from build123d import *

# Parameters (mm, degrees)
SALIENTE_EXTRUIR1_DEPTH = 8
CROQUIS2_R              = 10
CORTAR_EXTRUIR1_DEPTH   = 29.91366459
REDONDEO1_R             = 2
CROQUIS3_R              = 1.5
CORTAR_EXTRUIR2_DEPTH   = 30.159046624


with BuildPart() as part:
    # Croquis1 → Saliente-Extruir1 (new body)
    with BuildSketch(Plane.XY):
        with BuildLine():
            Line((-24, -0.5), (-13.99106858, -0.5))
            ThreePointArc((-13.99106858, -0.5), (0, 14), (13.99106858, -0.5))
            Line((13.99106858, -0.5), (24, -0.5))
            Line((24, -0.5), (24, -4.5))
            Line((24, -4.5), (13.257073584, -4.5))
            ThreePointArc((13.257073584, -4.5), (0, -14), (-13.257073584, -4.5))
            Line((-13.257073584, -4.5), (-24, -4.5))
            Line((-24, -4.5), (-24, -0.5))
        make_face()
    extrude(amount=SALIENTE_EXTRUIR1_DEPTH)

    # Croquis2 → Cortar-Extruir1 (cut, through all)
    with BuildSketch(Plane.XY.offset(8)):
        Circle(CROQUIS2_R)
    extrude(amount=-CORTAR_EXTRUIR1_DEPTH, mode=Mode.SUBTRACT)

    # Redondeo1
    redondeo1_edges = [part.edges().sort_by_distance(p)[0] for p in [
        (24, -2.5, 8),
        (-24, -2.5, 8),
        (-24, -2.5, 0),
        (24, -2.5, 0),
    ]]
    fillet(redondeo1_edges, radius=REDONDEO1_R)

    # Croquis3 → Cortar-Extruir2 (cut, through all)
    with BuildSketch(Plane(origin=(0, -0.5, 0), x_dir=(1, 0, 0), z_dir=(0, 1, 0))):
        with Locations(Location((-17.99553429, -4, 0), (0, 0, 270))):
            Circle(CROQUIS3_R)
        with Locations(Location((17.99553429, -4, 0), (0, 0, 270))):
            Circle(CROQUIS3_R)
    extrude(amount=-CORTAR_EXTRUIR2_DEPTH, mode=Mode.SUBTRACT)


solid = part.part
CAD build for the part. Positions are in the model's coordinates, mm. A direction names the side the tool comes from. Round coordinates to 2 decimals unless told otherwise and drop trailing zeros. Loops run counter-clockwise (first coordinate to the right, second up) from the corner with the lowest first, then second, coordinate; pieces in that order, holes last.
(1) Cut at B-B (x = 0). Give the cut face in (y, z), plus the area to 3 significant figures.
(2) Two-plate mould, pull along Z, no slides. Class faces 1 (the cylindrical face through (-19.326, -2.472, 4.692)), 2 (the cylindrical face through (23.4, -2.53, 0.57)), 3 (the flat face through (0.1, -10.3, 8)): +Z half, -Z half, draft (parallel to the pull), parting line (faces both ways), or undercut.
(3) Which spindle directions (+Z, -Z, +X, -X, +Y, -Y) get a long thin tool onto all of the face, cutting with end or side? Do faces 4 (the flat face through (-20, -4.5, 4)), 5 (the flat face through (20, -0.5, 4)), 6 (the flat face through (20, -4.5, 4)). Say none if no direction does.
(4) Cut at A-A (z = 4). Give the cut face in (x, y), plus the area to 3 significant figures.
(5) Drop flat-ended pins along their axis: pin 1 (3 mm diameter, centred on x = -1.5, z = 2.5, fed in from -Y); pin 2 (2 mm diameter, centred on x = 8.5, z = 1, fed in from +Y); pin 3 (2.5 mm diameter, centred on x = -17, z = 4, fed in from +Y); pin 4 (2 mm diameter, centred on y = -11, z = 6, fed in from -X). Give the stop position or say it passes through.
(6) Cut at D-D (x = 15.5). Give the cut face in (y, z), plus the area to 3 significant figures.
(7) Wall check: line 1 along X through (y, z) = (-2.45, 4); line 2 along X through (y, z) = (-3.25, 4); line 3 along Y through (x, z) = (20, 5). Give the ranges that are in metal, low to high.
Findings below:
1. outline: (-14, 0) - (-10, 0) - (-10, 8) - (-14, 8) - close; (10, 0) - (14, 0) - (14, 8) - (10, 8) - close
1. area: 64.0 mm2
2. face 1: undercut
2. face 2: -Z half
2. face 3: +Z half
3. face 4: +Z, -Z, -X, -Y
3. face 5: +Z, -Z, +X, +Y
3. face 6: +Z, -Z, +X, -Y
4. outline: (-24, -4.5) - (-19.5, -4.5) - (-19.5, -0.5) - (-24, -0.5) - close; (-16.5, -4.5) - (-13.26, -4.5) arc R14 ccw to (13.26, -4.5) - (16.5, -4.5) - (16.5, -0.5) - (13.99, -0.5) arc R14 ccw (long way) to (-13.99, -0.5) - (-16.5, -0.5) - close; (19.5, -4.5) - (24, -4.5) - (24, -0.5) - (19.5, -0.5) - close; hole circle Ø20 at (0, 0)
4. area: 360 mm2
5. pin 1: stops at y = -14
5. pin 2: stops at y = 11.82
5. pin 3: stops at y = -0.5
5. pin 4: stops at x = -9.8
6. outline: (-4.5, 0) - (-0.5, 0) - (-0.5, 8) - (-4.5, 8) - close
6. area: 32.0 mm2
7. line 1: x = -24 to -19.5, -16.5 to -9.7, 9.7 to 16.5, 19.5 to 24
7. line 2: x = -24 to -19.5, -16.5 to -9.46, 9.46 to 16.5, 19.5 to 24
7. line 3: y = -4.5 to -0.5
